Input: part model. Units: mm. Frame: model coordinates. A direction names the side the tool comes from. Coordinates: 2 decimals unless noted, no trailing zeros. Order: outer loops, then holes, each group sorted by start corner. A loop starts at its lowest first (then second) coordinate and runs counter-clockwise, first axis right, second up. Notation, with made-up numbers: (-21, -8.5) -> (30, -8.5) arc R12 cw to (30, 8.5) -> close; hole circle Ø6 at (1.25, -15.75). An arc over 180 degrees is marked (long way). Answer as CSV lines item,"result".
from build123d import *

# Parameters (mm, degrees)
BOSS_EXTRUDE1_DEPTH = 6.35


with BuildPart() as part:
    # Sketch2 → Boss-Extrude1 (new body)
    with BuildSketch(Plane(origin=(0, 0, 0), x_dir=(0, 0, -1), z_dir=(1, 0, 0))):
        with BuildLine():
            Line((14.859, 55.118), (14.859, 42.418))
            Line((14.859, 42.418), (21.209, 42.418))
            Line((21.209, 42.418), (21.209, 55.118))
            Line((21.209, 55.118), (27.559, 55.118))
            Line((27.559, 55.118), (27.559, 36.068))
            Line((27.559, 36.068), (36.068, 36.068))
            Line((36.068, 36.068), (36.068, 5.08))
            ThreePointArc((36.068, 5.08), (34.580102448, 1.487897552), (30.988, 0))
            Line((30.988, 0), (5.08, 0))
            ThreePointArc((5.08, 0), (1.487897552, 1.487897552), (0, 5.08))
            Line((0, 5.08), (0, 36.068))
            Line((0, 36.068), (8.509, 36.068))
            Line((8.509, 36.068), (8.509, 55.118))
            Line((8.509, 55.118), (14.859, 55.118))
        make_face()
        with BuildLine():
            Line((11.43, 6.35), (24.638, 6.35))
            ThreePointArc((24.638, 6.35), (28.230102448, 7.837897552), (29.718, 11.43))
            Line((29.718, 11.43), (29.718, 24.638))
            ThreePointArc((29.718, 24.638), (28.230102448, 28.230102448), (24.638, 29.718))
            Line((24.638, 29.718), (11.43, 29.718))
            ThreePointArc((11.43, 29.718), (7.837897552, 28.230102448), (6.35, 24.638))
            Line((6.35, 24.638), (6.35, 11.43))
            ThreePointArc((6.35, 11.43), (7.837897552, 7.837897552), (11.43, 6.35))
        make_face(mode=Mode.SUBTRACT)
    extrude(amount=BOSS_EXTRUDE1_DEPTH)


solid = part.part
1. Cut plane C-C (x = 1.75). Return the cut outline in (y, z), plus the area to 3 significant figures.
Findings:
outline,"(0, -30.99) arc R5.08 ccw to (5.08, -36.07) -> (36.07, -36.07) -> (36.07, -27.56) -> (55.12, -27.56) -> (55.12, -21.21) -> (42.42, -21.21) -> (42.42, -14.86) -> (55.12, -14.86) -> (55.12, -8.51) -> (36.07, -8.51) -> (36.07, 0) -> (5.08, 0) arc R5.08 ccw to (0, -5.08) -> close; hole (6.35, -24.64) arc R5.08 ccw to (11.43, -29.72) -> (24.64, -29.72) arc R5.08 ccw to (29.72, -24.64) -> (29.72, -11.43) arc R5.08 ccw to (24.64, -6.35) -> (11.43, -6.35) arc R5.08 ccw to (6.35, -11.43) -> close"
area,"1,050 mm2"
2. Contact query for flat-ended pins moving along their axis: pin 1 (1.9 mm diameter, centred on x = 3.5, y = 49, fed in from -Z); pin 2 (1.9 mm diameter, centred on x = 3, y = 49, fed in from +Z); pin 3 (3 mm diameter, centred on x = 2.5, z = -19.5, fed in from +Y); pin 4 (10 mm diameter, centred on y = 25.5, z = -20.5, fed in from -X). Output: stop coordinate, or through.
Findings:
pin 1,"stops at z = -27.56"
pin 2,"stops at z = -8.51"
pin 3,"stops at y = 42.42"
pin 4,"stops at x = 0"
3. Cut plane B-B (z = -19). Return the cut outline in (x, y).
Findings:
outline,"(0, 0) -> (6.35, 0) -> (6.35, 6.35) -> (0, 6.35) -> close; (0, 29.72) -> (6.35, 29.72) -> (6.35, 42.42) -> (0, 42.42) -> close"
4. Cut plane D-D (y = 37). Return the cut outline in (x, z), plus the area to 3 significant figures.
Findings:
outline,"(0, -27.56) -> (6.35, -27.56) -> (6.35, -8.51) -> (0, -8.51) -> close"
area,"121 mm2"
5. Ray query, line 1 along Y through (x, z) = (0.5, -23.5); line 2 along Y through (x, z) = (3.5, -17.5); line 3 along Z through (x, y) = (2.5, 46). Return the intervals inside material, ascending.
Findings:
line 1,"y = 0 to 6.35, 29.72 to 55.12"
line 2,"y = 0 to 6.35, 29.72 to 42.42"
line 3,"z = -27.56 to -21.21, -14.86 to -8.51"
6. Cut plane A-A (y = 16.5). Return the cut outline in (x, z).
Findings:
outline,"(0, -36.07) -> (6.35, -36.07) -> (6.35, -29.72) -> (0, -29.72) -> close; (0, -6.35) -> (6.35, -6.35) -> (6.35, 0) -> (0, 0) -> close"
7. Reachability of faces 1 (the face through (3.13, 28.19, -28.27)), 2 (the face through (3, 36.068, -32)), 3 (the face through (3, 45, -8.509)), 4 (the face through (3, 49, -14.859)) from +Z, -Z, +X, -X, +Y, -Y: full face, straight path, thin tool, end or side. Return the list, or none.
Findings:
face 1,"+X, -X"
face 2,"-Z, +X, -X, +Y"
face 3,"+Z, +X, -X, +Y"
face 4,"+X, -X, +Y"
8. Mould query, pull axis Z, two halves, no side actions, for faces 5 (the face through (3, 18, -6.35)), 6 (the face through (3, 49, -21.209)), 7 (the face through (3.131, 1.449, -1.528)), 8 (the face through (3, 36.068, -4)). Classes: released by +Z, released by -Z, zero draft, split by the parting line, or undercut.
Findings:
face 5,"undercut"
face 6,"undercut"
face 7,"released by +Z"
face 8,"zero draft"
